Here's the drawing with two shaded views (mm, measured from the low corner). I have some questions. A direction names the side the tool comes from. Round coordinates to 2 decimals unless told otherwise and drop trailing zeros. Write each loop counter-clockwise with the first axis right and the second up, starting at its lowest first coordinate (ties: lowest second). Pieces come first, ordered by that corner, then holes. Notation, with made-up numbers: M 87,77.25 L 106,77.25 A28 ccw 106,106.25 Z; hole C 10.25,71 d5. An arc over 180 degrees is marked long. Answer as a JSON object with one key per item and string values. Group by question number.
1) I'm going to push flat-ended pins straight in: pin 1 Ø1.2 at (y, z) = (4.5, 7.5) entering from +X; pin 2 Ø2.5 at (x, z) = (35, 5) entering from +Y; pin 3 Ø6.5 at (x, z) = (5, 5) entering from +Y; pin 4 Ø2 at (y, z) = (5.5, 4) entering from -X. Where does each tip first touch, or does it pass through?
2) Please list where these lines run through material, in increasing order: L1, parallel to Z at x = 5, y = 2.7; L2, parallel to X at y = 8, z = 15; L3, parallel to Y at x = 18.5, z = 17.25. Write a range as [from, to].
3) Suppose I cut it at B-B, the plane y = 5. Write out the boundary of the cut face in (x, z).
4) If we mould it in two halves opening along X, with no side actions, what happens to the marked faces 3, 4, 5 and 6? For each: +X half, -X half, draft (parallel to the pull), parting line (faces both ways), or undercut.
5) Suppose I cut it at D-D, the plane x = 35. Write out the boundary of the cut face in (y, z), and give its area (3 significant figures).
6) On a 3-axis mill with a long thin cutter (end or side, diameter ignored), from which of +Z, -Z, +X, -X, +Y, -Y can I reach the whole of each face in a straight line? I mean the marked faces 1 and 2. Say none if no direction works.
7) Suppose I cut it at A-A, the plane z = 5. State how many separate pieces and enclosed holes the cut face has, and give its area (3 significant figures).
8) Suppose I cut it at C-C, the plane y = 9.5. Write out the boundary of the cut face in (x, z), and give its area (3 significant figures).
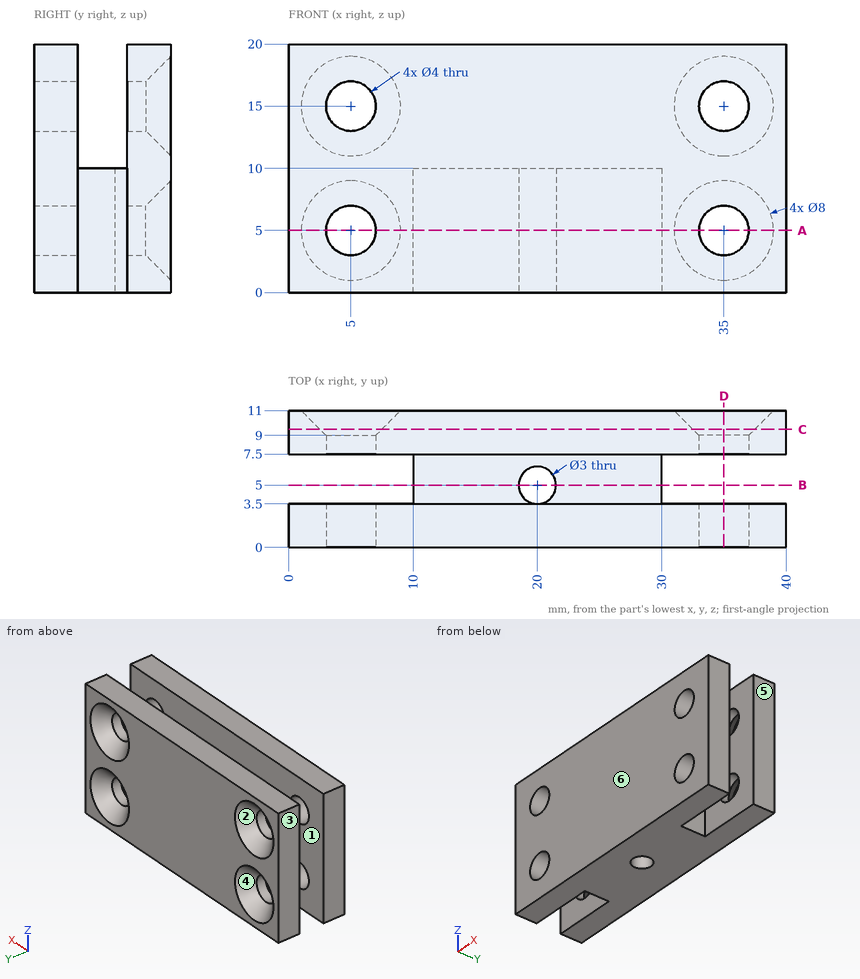
Results:
{
 "1": {"pin 1": "x = 30", "pin 2": "through", "pin 3": "y = 10.25", "pin 4": "x = 10"},
 "2": {"L1": "[0, 3], [7, 13], [17, 20]", "L2": "[0, 3], [7, 33], [37, 40]", "L3": "[0, 3.5], [7.5, 11]"},
 "3": {"outline": "M 10,0 L 18.5,0 L 18.5,10 L 10,10 Z; M 21.5,0 L 30,0 L 30,10 L 21.5,10 Z"},
 "4": {"face 3": "-X half", "face 4": "undercut", "face 5": "+X half", "face 6": "draft"},
 "5": {"outline": "M 0,0 L 3.5,0 L 3.5,3 L 0,3 Z; M 0,7 L 3.5,7 L 3.5,13 L 0,13 Z; M 0,17 L 3.5,17 L 3.5,20 L 0,20 Z; M 7.5,0 L 11,0 L 11,1 L 9,3 L 7.5,3 Z; M 7.5,7 L 9,7 L 11,9 L 11,11 L 9,13 L 7.5,13 Z; M 7.5,17 L 9,17 L 11,19 L 11,20 L 7.5,20 Z", "area": "76.0 mm^2"},
 "6": {"face 1": "+Z", "face 2": "+Y"},
 "7": {"separate pieces": "5", "enclosed holes": "1", "area": "289 mm^2"},
 "8": {"outline": "M 0,0 L 40,0 L 40,20 L 0,20 Z; hole C 5,5 d5; hole C 5,15 d5; hole C 35,5 d5; hole C 35,15 d5", "area": "721 mm^2"}
}
